from build123d import *

# Parameters (mm, degrees)
BOSS_EXTRUDE1_DEPTH     = 21
SKETCH5_W               = 6.2
SKETCH5_H               = 6.2
CUT_EXTRUDE1_DEPTH      = 5
CUT_EXTRUDE2_DEPTH      = 28.364438602
CUT_EXTRUDE2_DEPTH_BACK = 28.364438602
SKETCH9_W               = 24.284850455
SKETCH9_H               = 22.464844075
CUT_EXTRUDE3_DEPTH      = 3
SKETCH10_W              = 31.815901763
SKETCH10_H              = 21.67332365
CUT_EXTRUDE4_DEPTH      = 4


with BuildPart() as part:
    # Sketch3 → Boss-Extrude1 (new body)
    with BuildSketch(Plane(origin=(0, 0, 0), x_dir=(0, 0, -1), z_dir=(1, 0, 0))):
        with BuildLine():
            Line((-12.75, -9.5), (12.75, -9.5))
            ThreePointArc((12.75, -9.5), (14.164213562, -8.914213562), (14.75, -7.5))
            Line((14.75, -7.5), (14.75, 7.5))
            ThreePointArc((14.75, 7.5), (14.164213562, 8.914213562), (12.75, 9.5))
            Line((12.75, 9.5), (-12.75, 9.5))
            ThreePointArc((-12.75, 9.5), (-14.164213562, 8.914213562), (-14.75, 7.5))
            Line((-14.75, 7.5), (-14.75, -7.5))
            ThreePointArc((-14.75, -7.5), (-14.164213562, -8.914213562), (-12.75, -9.5))
        make_face()
    extrude(amount=BOSS_EXTRUDE1_DEPTH)

    # Sketch5 → Cut-Extrude1 (cut)
    with BuildSketch(Plane(origin=(0, 9.5, 0), x_dir=(1, 0, 0), z_dir=(0, 1, 0))):
        with Locations((3.1, 0)):
            Rectangle(SKETCH5_W, SKETCH5_H)
    extrude(amount=-CUT_EXTRUDE1_DEPTH, mode=Mode.SUBTRACT)

    # Sketch7 → Cut-Extrude2 (cut, two sides: drawn at the far end of the back side and taken through both)
    with BuildSketch(Plane.ZY.offset(-CUT_EXTRUDE2_DEPTH_BACK)):
        with BuildLine():
            Line((-11.147623693, -8.072928754), (11.147623693, -8.072928754))
            ThreePointArc((11.147623693, -8.072928754), (12.561837255, -7.487142316), (13.147623693, -6.072928754))
            Line((13.147623693, -6.072928754), (13.147623693, 0.135263404))
            ThreePointArc((13.147623693, 0.135263404), (12.561837255, 1.549476966), (11.147623693, 2.135263404))
            Line((11.147623693, 2.135263404), (-11.147623693, 2.135263404))
            ThreePointArc((-11.147623693, 2.135263404), (-12.561837255, 1.549476966), (-13.147623693, 0.135263404))
            Line((-13.147623693, 0.135263404), (-13.147623693, -6.072928754))
            ThreePointArc((-13.147623693, -6.072928754), (-12.561837255, -7.487142316), (-11.147623693, -8.072928754))
        make_face()
    extrude(amount=CUT_EXTRUDE2_DEPTH + CUT_EXTRUDE2_DEPTH_BACK, mode=Mode.SUBTRACT)

    # Sketch9 → Cut-Extrude3 (cut)
    with BuildSketch(Plane(origin=(0, 9.5, 0), x_dir=(1, 0, 0), z_dir=(0, 1, 0))):
        with Locations((12.142425228, 0.007615305)):
            Rectangle(SKETCH9_W, SKETCH9_H)
    extrude(amount=-CUT_EXTRUDE3_DEPTH, mode=Mode.SUBTRACT)

    # Sketch10 → Cut-Extrude4 (cut)
    with BuildSketch(Plane(origin=(21, 0, 0), x_dir=(0, 0, -1), z_dir=(1, 0, 0))):
        with Locations((-0.011194899, 0.447795943)):
            Rectangle(SKETCH10_W, SKETCH10_H)
    extrude(amount=-CUT_EXTRUDE4_DEPTH, mode=Mode.SUBTRACT)


solid = part.part
Build history of the part. All positions in model axes, mm. A direction names the side the tool comes from. Round coordinates to 2 decimals unless told otherwise and drop trailing zeros. Write each loop counter-clockwise with the first axis right and the second up, starting at its lowest first coordinate (ties: lowest second). Pieces come first, ordered by that corner, then holes. Notation, with made-up numbers: (-23.75, -36) -> (29.25, -36) arc R17 ccw to (29.25, -11) -> close; hole circle Ø7 at (-9.75, 1). An arc over 180 degrees is marked (long way). Use one line per item in the form item = value.
Q1. Band-saw the part on A-A, the plane y = -3.25. Write the cut outline in (x, z), then the cut area to 3 significant figures.
Conclusion:
outline = (0, -14.75) -> (17, -14.75) -> (17, -13.15) -> (0, -13.15) -> close; (0, 13.15) -> (17, 13.15) -> (17, 14.75) -> (0, 14.75) -> close
area = 54.5 mm²
Q2. Drill centre lines: L1, parallel to Y at x = 4.5, z = 7; L2, parallel to Z at x = 1, y = 0; L3, parallel to Z at x = 1, y = 1. Where is each one in solid material? Low to high.
Conclusion:
L1 = -9.5 to -8.07, 2.14 to 6.5
L2 = -14.75 to -13.15, 13.15 to 14.75
L3 = -14.75 to -12.95, 12.95 to 14.75
Q3. Band-saw the part on B-B, the plane z = 3.5. Write the cut outline in (x, y).
Conclusion:
outline = (0, -9.5) -> (17, -9.5) -> (17, -8.07) -> (0, -8.07) -> close; (0, 2.14) -> (17, 2.14) -> (17, 6.5) -> (0, 6.5) -> close
Q4. Drop flat-ended pins along their axis: P1, Ø1, axis at y = 5.5, z = -1.5, coming from the -X side; P2, Ø1.9, axis at x = 4.5, z = -0.5, coming from the +Y side. Give the stop position or say it passes through.
Conclusion:
P1 = 6.2
P2 = 4.5
Q5. Tool access for faces 1 (the flat face through (9, -3, 13.148)), 2 (the flat face through (8, 0, -14.75)), 3 (the flat face through (3, 4.5, 0)): list every direction of +Z, -Z, +X, -X, +Y, -Y with a clear straight run to the whole face (end or side of a thin tool).
Conclusion:
face_1 = +X, -X
face_2 = -Z, +X, -X, +Y, -Y
face_3 = -X, +Y
Q6. Two-plate mould, pull along Y, no slides. Class faces 4 (the flat face through (8, 6.5, 0)), 5 (the flat face through (8, -9.5, 0)), 6 (the cylindrical face through (8.62, -7.47, -12.58)), 7 (the flat face through (3, 6, -3.1)): released by +Y, released by -Y, zero draft, split by the parting line, or undercut.
Conclusion:
face_4 = released by +Y
face_5 = released by -Y
face_6 = undercut
face_7 = zero draft
Q7. Band-saw the part on D-D, the plane z = -0.75. Write the cut outline in (x, y).
Conclusion:
outline = (0, -9.5) -> (17, -9.5) -> (17, -8.07) -> (0, -8.07) -> close; (0, 2.14) -> (17, 2.14) -> (17, 6.5) -> (6.2, 6.5) -> (6.2, 4.5) -> (0, 4.5) -> close
Q8. Band-saw the part on C-C, the plane x = 3. Write the cut outline in (y, z).
Conclusion:
outline = (-9.5, -12.75) arc R2 ccw to (-7.5, -14.75) -> (7.5, -14.75) arc R2 ccw to (9.5, -12.75) -> (9.5, -11.24) -> (6.5, -11.24) -> (6.5, -3.1) -> (4.5, -3.1) -> (4.5, 3.1) -> (6.5, 3.1) -> (6.5, 11.22) -> (9.5, 11.22) -> (9.5, 12.75) arc R2 ccw to (7.5, 14.75) -> (-7.5, 14.75) arc R2 ccw to (-9.5, 12.75) -> close; hole (-8.07, -11.15) arc R2 ccw to (-6.07, -13.15) -> (0.14, -13.15) arc R2 ccw to (2.14, -11.15) -> (2.14, 11.15) arc R2 ccw to (0.14, 13.15) -> (-6.07, 13.15) arc R2 ccw to (-8.07, 11.15) -> close
